Work out the finished part from the listing and answer in its coordinate system (mm). A direction names the side the tool comes from. Round coordinates to 2 decimals unless told otherwise and drop trailing zeros. Loops run counter-clockwise (first coordinate to the right, second up) from the corner with the lowest first, then second, coordinate; pieces in that order, holes last. Notation, with made-up numbers: (43.25, 7) -> (71.25, 7) arc R29 ccw to (71.25, 36) -> close; hole circle Ø5 at (-11, 46.25). An arc over 180 degrees is marked (long way). Use one line per item in the form item = value.
```python
from build123d import *

# Parameters (mm, degrees)
F1_DEPTH  = 29.2991027236
F2_DEPTH  = 40.9627631307
F3_DEPTH  = 68.8303261995
F4_T      = -2.54
F5_W      = 95.6771153452
F5_H      = 29.2991027236
F5_R      = 8.1039957671
F6_DEPTH  = 25
F7_R      = 8.5249443269
F8_DEPTH  = 25
F10_DEPTH = 100


with BuildPart() as f1:
    # F0 (on Top) → F1 (new body)
    with BuildSketch(Plane.XY):
        Polygon((17.0515403152, -60.0674971938), (0, 34.0778976679), (-59.2823252082, 9.1290585697), align=None)
    extrude(amount=-F1_DEPTH)

    # F2 (add): a face of the model
    f2_faces = [f1.faces().sort_by_distance(p)[0] for p in [
        (-29.6411626041, 21.6034781188, -14.6495513618),
    ]]
    extrude(f2_faces, amount=F2_DEPTH)

    # F3 (add): a face of the model
    f3_faces = [f1.faces().sort_by_distance(p)[0] for p in [
        (-67.2269849041, 28.0068066647, -14.6495513618),
    ]]
    extrude(f3_faces, amount=F3_DEPTH)

    # F4
    f4_openings = [f1.faces().sort_by_distance(p)[0] for p in [
        (-130.668094, 1.307752, -14.649551),
    ]]
    offset(amount=F4_T, openings=f4_openings, kind=Kind.INTERSECTION)

    # F5 (on face) → F6 (join)
    with BuildSketch(Plane(origin=(5.9761205036, 1.0823902735, 0), x_dir=(-0.1782196323, 0.983990733, 0), z_dir=(0.983990733, 0.1782196323, 0))):
        with Locations((-14.3062221666, -14.6495513618)):
            Rectangle(F5_W, F5_H)
        with Locations((-26.3812504709, -13.2899768651)):
            Circle(F5_R, mode=Mode.SUBTRACT)
    extrude(amount=F6_DEPTH)

    # F7 (on face) → F8 (join)
    with BuildSketch(Plane.XY):
        with Locations((-45.2117063105, 26.2168720365)):
            Circle(F7_R)
    extrude(amount=F8_DEPTH)

    # F9 (on face) → F10 (join)
    with BuildSketch(Plane.XY.offset(25)):
        with BuildLine():
            ThreePointArc((-64.3323721087, 36.3062107036), (-56.9744432535, 36.3138053878), (-53.293284687, 29.9429148436))
            ThreePointArc((-53.293284687, 29.9429148436), (-58.8077923617, 22.8230389836), (-67.0805371507, 26.3817073875))
            ThreePointArc((-67.0805371507, 26.3817073875), (-64.7228255119, 16.131982496), (-57.7273939024, 8.2783463241))
            ThreePointArc((-57.7273939024, 8.2783463241), (-50.3687668703, 12.7783108002), (-44.8766799987, 19.4293298107))
            ThreePointArc((-44.8766799987, 19.4293298107), (-51.7516634602, 28.0640137679), (-41.3753042644, 31.8262384388))
            ThreePointArc((-41.3753042644, 31.8262384388), (-41.3686098103, 32.1676324461), (-41.3663781986, 32.5090847909))
            ThreePointArc((-41.3663781986, 32.5090847909), (-42.4957862059, 40.1072719094), (-45.7863536257, 47.0484660424))
            ThreePointArc((-45.7863536257, 47.0484660424), (-56.5176025345, 44.194923272), (-64.3323721087, 36.3062107036))
        make_face()
        with BuildLine():
            ThreePointArc((-67.0805371507, 26.3817073875), (-67.7337027998, 31.9053183776), (-64.3323721087, 36.3062107036))
            ThreePointArc((-64.3323721087, 36.3062107036), (-56.5176025345, 44.194923272), (-45.7863536257, 47.0484660424))
            ThreePointArc((-45.7863536257, 47.0484660424), (-92.4558918977, 40.198539381), (-57.7273939024, 8.2783463241))
            ThreePointArc((-57.7273939024, 8.2783463241), (-64.7228255119, 16.131982496), (-67.0805371507, 26.3817073875))
        make_face()
        with BuildLine():
            ThreePointArc((-24.706517752, 25.8585140109), (-30.874012332, 40.8031915547), (-45.7863536257, 47.0484660424))
            ThreePointArc((-45.7863536257, 47.0484660424), (-42.4957862059, 40.1072719094), (-41.3663781986, 32.5090847909))
            ThreePointArc((-41.3663781986, 32.5090847909), (-41.3686098103, 32.1676324461), (-41.3753042644, 31.8262384388))
            ThreePointArc((-41.3753042644, 31.8262384388), (-39.2011150693, 29.3879546634), (-38.4159008325, 26.2168720365))
            ThreePointArc((-38.4159008325, 26.2168720365), (-40.2893214342, 21.5314585835), (-44.8766799987, 19.4293298107))
            ThreePointArc((-44.8766799987, 19.4293298107), (-50.3687668703, 12.7783108002), (-57.7273939024, 8.2783463241))
            ThreePointArc((-57.7273939024, 8.2783463241), (-35.9385388446, 7.153965382), (-24.706517752, 25.8585140109))
        make_face()
    extrude(amount=-F10_DEPTH)


solid = f1.part
```
(1) Consider L1, parallel to Z at x = -11.5, y = -17.5; L2, parallel to Y at x = -90, z = -11; L3, parallel to X at y = 40.5, z = -12.5. Determine where each line is inside the solid, lowest interval first.
Completed:
L1 = -29.3 to -26.76, -2.54 to 0
L2 = -3.8 to -1.04, 19.25 to 45.77
L3 = -92.36 to -30.58, -5.46 to -2.7
(2) Given P1, Ø2, axis at y = 47.5, z = -12.5, coming from the +X side; P2, Ø3, axis at x = -90.5, z = -24.5, coming from the -Y side; P3, Ø4.5, axis at x = -59.5, y = 28.5, coming from the +Z side; P4, Ø23.5, axis at x = -60.65, y = 29.94, coming from the +Z side, each flat-ended and moving along its own axis, determine where each tip first touches the part or whether it passes through.
Completed:
P1 = -5.23
P2 = -4.64
P3 = 0
P4 = 25
(3) For faces 1 (the flat face through (-97.281, -4.107, -14.48)), 2 (the flat face through (12.128, 36.274, -14.855)), 3 (the flat face through (-18, 15, -26.759)), 4 (the flat face through (29.18, -57.87, -14.85)), 5 (the flat face through (-61, 30, -29.299)), determine the directions among +Z, -Z, +X, -X, +Y, -Y from which every point of the face is accessible in a straight line to the end or side of a thin tool.
Completed:
face_1 = -X
face_2 = +Z, -Z, +Y
face_3 = none
face_4 = +Z, -Z, +X, -Y
face_5 = -Z
(4) Find section C-C, the plane z = -55. Write down the section's boundary in (x, y), then the cut area to 3 significant figures.
Completed:
outline = (-57.73, 8.28) arc R21.19 ccw (long way) to (-45.79, 47.05) arc R26.12 ccw (long way) to start; hole circle Ø14.71 at (-60.65, 29.94); hole circle Ø13.59 at (-45.21, 26.22)
area = 2,520 mm2
(5) Find section B-B, the plane x = -33. Write down the section's boundary in (y, z), then the cut area to 3 significant figures.
Completed:
outline = (-14.7, -29.3) -> (9.04, -29.3) -> (9.04, -75) -> (42.67, -75) -> (42.67, -29.3) -> (64.63, -29.3) -> (64.63, 0) -> (42.67, 0) -> (42.67, 25) -> (9.04, 25) -> (9.04, 0) -> (-14.7, 0) -> close; hole (-11.27, -26.76) -> (9.04, -26.76) -> (9.04, -2.54) -> (-11.27, -2.54) -> close; hole (42.67, -26.76) -> (61.88, -26.76) -> (61.88, -2.54) -> (42.67, -2.54) -> close
area = 3,740 mm2
(6) Find section A-A, the plane y = -0.5. Write down the section's boundary in (x, z).
Completed:
outline = (-129.91, -29.3) -> (-82.16, -29.3) -> (-82.16, 0) -> (-129.91, 0) -> (-129.91, -2.54) -> (-88.71, -2.54) -> (-88.71, -26.76) -> (-129.91, -26.76) -> close; (-48.66, -29.3) -> (31.67, -29.3) -> (31.67, 0) -> (-48.66, 0) -> close; hole (-44.88, -26.76) -> (3.68, -26.76) -> (3.68, -2.54) -> (-44.88, -2.54) -> close
(7) Find section D-D, the plane x = -83.5. Write down the section's boundary in (y, z), then the cut area to 3 significant figures.
Completed:
outline = (-1.06, -29.3) -> (11.87, -29.3) -> (11.87, -75) -> (53.15, -75) -> (53.15, 25) -> (11.87, 25) -> (11.87, 0) -> (-1.06, 0) -> close; hole (1.69, -26.76) -> (11.87, -26.76) -> (11.87, -2.54) -> (1.69, -2.54) -> close
area = 4,260 mm2
(8) For a pull along X with two mould halves and no side action, classify faces 6 (the cylindrical face through (-48.69, 50.65, -14.48)), 7 (the flat face through (-4, 4, 0)), 8 (the flat face through (-115.311, 29.992, -14.444)), 9 (the flat face through (33.245, -9.198, -14.444)) as +X half, -X half, draft (parallel to the pull), parting line (faces both ways), or undercut.
Completed:
face_6 = undercut
face_7 = draft
face_8 = -X half
face_9 = +X half
